```python
from build123d import *

# Parameters (mm, degrees)
SKETCH1_R              = 2.5
BOSS_EXTRUDE1_DEPTH    = 7
CUT_EXTRUDE1_START     = -40
CUT_EXTRUDE1_OUTLINE_W = 34.803170534
CUT_EXTRUDE1_OUTLINE_H = 6
CUT_EXTRUDE1_DEPTH     = 46.239041119
FILLET1_R              = 3


# Read off the part's stored shape, not the designer's step: Cut-Extrude1
with BuildPart() as part:
    # Sketch1 → Boss-Extrude1 (new, symmetric)
    with BuildSketch(Plane(origin=(0, 0, 0), x_dir=(1, 0, 0), z_dir=(0, 1, 0))):
        with BuildLine():
            Line((-16.647024265, 22.786117759), (-20.826247522, -0.869862938))
            ThreePointArc((-20.826247522, -0.869862938), (-28.357947563, -6.139919341), (-33.628003966, 1.391780701))
            Line((-33.628003966, 1.391780701), (-21.433938056, 70.414795281))
            Line((-21.433938056, 70.414795281), (-5, 90))
            Line((-5, 90), (0, 90))
            Line((0, 90), (0, 88.40012962))
            Line((0, 88.40012962), (-2, 86.400129391))
            Line((-2, 86.400129391), (0, 84.40012962))
            Line((0, 84.40012962), (-2, 82.400129391))
            Line((-2, 82.400129391), (0, 80.40012962))
            Line((0, 80.40012962), (-2, 78.400129391))
            Line((-2, 78.400129391), (0, 76.40012962))
            Line((0, 76.40012962), (0, 75))
            ThreePointArc((0, 75), (-7.146428929, 57.5), (0, 40))
            Line((0, 40), (-2, 38.00000006))
            Line((-2, 38.00000006), (0, 36))
            Line((0, 36), (-2, 34.00000006))
            Line((-2, 34.00000006), (0, 32))
            Line((0, 32), (-2, 30.353333333))
            Line((-2, 30.353333333), (-5.059793432, 30.89389684))
            ThreePointArc((-5.059793432, 30.89389684), (-12.532584877, 29.23980138), (-16.647024265, 22.786117759))
        make_face()
        with Locations(Location((-25.75, 0, 0), (0, 0, 270))):
            Circle(SKETCH1_R, mode=Mode.SUBTRACT)
        with Locations(Location((-20.45, 30, 0), (0, 0, 270))):
            Circle(SKETCH1_R, mode=Mode.SUBTRACT)
    extrude(amount=BOSS_EXTRUDE1_DEPTH, both=True)

    # Cut-Extrude1 outline → Cut-Extrude1 (cut)
    with BuildSketch(Plane.XY.offset(CUT_EXTRUDE1_START)):
        with Locations((-17.401585267, 0)):
            Rectangle(CUT_EXTRUDE1_OUTLINE_W, CUT_EXTRUDE1_OUTLINE_H)
    extrude(amount=CUT_EXTRUDE1_DEPTH, mode=Mode.SUBTRACT)

    # Fillet1
    fillet1_edges = [part.edges().sort_by_distance(p)[0] for p in [
        (-21.433938056, 0, -70.414795281),
        (-5, 0, -90),
    ]]
    fillet(fillet1_edges, radius=FILLET1_R)


solid = part.part
```
Part model, mm, in its own coordinate system. A direction names the side the tool comes from. Round coordinates to 2 decimals unless told otherwise and drop trailing zeros. Loops run counter-clockwise (first coordinate to the right, second up) from the corner with the lowest first, then second, coordinate; pieces in that order, holes last.
Item 1: Drill centre lines: line 1 (Y direction, x = -16, z = -33); line 2 (X direction, y = -5.7, z = -30); line 3 (Z direction, x = -3, y = 3.75). Where is each one in solid material? Low to high.
Item 2: Cut at D-D, the plane x = -11. Give the cut face in (y, z).
Item 3: 3-axis set-ups, long thin cutter, end or side, ignore diameter. For faces 1 (the face through (-20.34, 4.972, -32.498)), 2 (the face through (-21, 3, -22)), 3 (the face through (-1, -5, -39)): which of +Z, -Z, +X, -X, +Y, -Y reach the whole face in a straight line?
Item 4: Mould opens along X. For faces 4 (the face through (-3.51, 5.03, -30.62)), 5 (the face through (-28.217, 5.028, 6.163)), 6 (the face through (-2, 0, -90)), 7 (the face through (-7.145, 0.098, -57.771)) say: +X half, -X half, draft (parallel to the pull), parting line (faces both ways), or undercut.
Item 5: Cut at A-A, the plane z = -13. Give the cut face in (x, y).
Item 6: Cut at B-B, the plane x = -25.75. Give the cut face in (y, z), then the cut area to 3 significant figures.
Item 7: Cut at C-C, the plane z = 0. Give the cut face in (x, y).
Item 8: Drop flat-ended pins along their axis: P1, Ø5, axis at x = -9, y = 5.5, coming from the +Z side; P2, Ø3, axis at x = -17, z = -17.5, coming from the +Y side; P3, Ø6, axis at y = -3.5, z = -49, coming from the -X side; P4, Ø1.8, axis at x = -15, y = -1, coming from the +Z side. Give the stop position or say it passes through.
A:
1. line 1: y = -7 to -3, 3 to 7
1. line 2: x = -28.57 to -22.95, -17.95 to -11.25
1. line 3: z = -90 to -71.29, -43.71 to -30.53
2. outline: (-7, -82.85) - (7, -82.85) - (7, -30.12) - (3, -30.12) - (3, -40) - (-3, -40) - (-3, -30.12) - (-7, -30.12) - close
3. face 1: +Y, -Y
3. face 2: +Z, +X, -X
3. face 3: +X, +Y, -Y
4. face 4: undercut
4. face 5: parting line
4. face 6: draft
4. face 7: +X half
5. outline: (-31.58, -7) - (-18.38, -7) - (-18.38, -3) - (-31.58, -3) - close; (-31.58, 3) - (-18.38, 3) - (-18.38, 7) - (-31.58, 7) - close
6. outline: (-7, -45.98) - (7, -45.98) - (7, -2.5) - (3, -2.5) - (3, -40) - (-3, -40) - (-3, -2.5) - (-7, -2.5) - close; (-7, 2.5) - (-3, 2.5) - (-3, 6.07) - (-7, 6.07) - close; (3, 2.5) - (7, 2.5) - (7, 6.07) - (3, 6.07) - close
6. area: 412 mm2
7. outline: (-33.72, -7) - (-28.25, -7) - (-28.25, -3) - (-33.72, -3) - close; (-33.72, 3) - (-28.25, 3) - (-28.25, 7) - (-33.72, 7) - close; (-23.25, -7) - (-20.67, -7) - (-20.67, -3) - (-23.25, -3) - close; (-23.25, 3) - (-20.67, 3) - (-20.67, 7) - (-23.25, 7) - close
8. P1: stops at z = -29.87
8. P2: stops at y = 7
8. P3: stops at x = -25.75
8. P4: stops at z = -40
